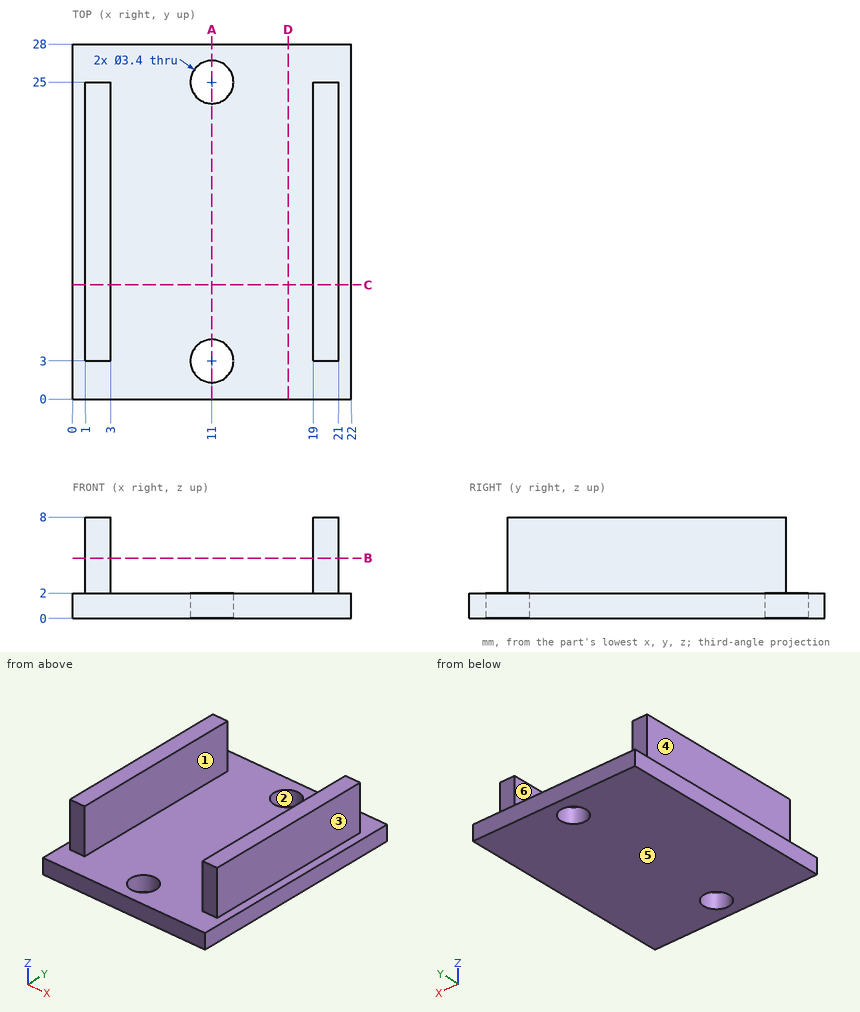
Verification items for this drawing (mm, ordinates from the low corner). A direction names the side the tool comes from. Round coordinates to 2 decimals unless told otherwise and drop trailing zeros. Order: outer loops, then holes, each group sorted by start corner. A loop starts at its lowest first (then second) coordinate and runs counter-clockwise, first axis right, second up.
1) Material ranges on line 1 (Y direction, x = 11, z = 0.7); line 2 (X direction, y = 10, z = 3); line 3 (Z direction, x = 18.5, y = 9), recorded low to high.
Geometry says:
line 1: y = 0 to 1.3, 4.7 to 23.3, 26.7 to 28
line 2: x = 1 to 3, 19 to 21
line 3: z = 0 to 2
2) Draft check along X on the marked faces 4, 5 and 6. Enter one of: +X half, -X half, draft (parallel to the pull), parting line (faces both ways), or undercut.
Geometry says:
face 4: -X half
face 5: draft
face 6: undercut
3) Tool access check on the marked faces 1, 2 and 3. Record the directions out of +Z, -Z, +X, -X, +Y, -Y that give a thin tool (end or side, any length) a straight path to the whole face; none if there is none.
Geometry says:
face 1: +Z, +Y, -Y
face 2: +Z, -Z
face 3: +Z, +X, +Y, -Y
4) Cross-section at D-D, the plane x = 17. Record the cut outline in (y, z).
Geometry says:
outline: (0, 0) - (28, 0) - (28, 2) - (0, 2) - close
5) Cross-section at A-A, the plane x = 11. Record the cut outline in (y, z), plus the area to 3 significant figures.
Geometry says:
outline: (0, 0) - (1.3, 0) - (1.3, 2) - (0, 2) - close; (4.7, 0) - (23.3, 0) - (23.3, 2) - (4.7, 2) - close; (26.7, 0) - (28, 0) - (28, 2) - (26.7, 2) - close
area: 42.4 mm2
6) Cross-section at C-C, the plane y = 9. Record the cut outline in (x, z), plus the area to 3 significant figures.
Geometry says:
outline: (0, 0) - (22, 0) - (22, 2) - (21, 2) - (21, 8) - (19, 8) - (19, 2) - (3, 2) - (3, 8) - (1, 8) - (1, 2) - (0, 2) - close
area: 68.0 mm2
7) Cross-section at B-B, the plane z = 4.75. Record the cut outline in (x, y).
Geometry says:
outline: (1, 3) - (3, 3) - (3, 25) - (1, 25) - close; (19, 3) - (21, 3) - (21, 25) - (19, 25) - close
8) Depth check by flat-ended pin: pin 1 (0.6 mm diameter, centred on x = 20, z = 6, fed in from +Y); pin 2 (4 mm diameter, centred on y = 11.5, z = 3.5, fed in from -X); pin 3 (3 mm diameter, centred on y = 12, z = 5, fed in from -X); pin 4 (4 mm diameter, centred on x = 4, z = 5, fed in from -Y). Enter the tip coordinate at first touch or a pass-through.
Geometry says:
pin 1: stops at y = 25
pin 2: stops at x = 0
pin 3: stops at x = 1
pin 4: stops at y = 3
